from build123d import *

# Parameters (mm, degrees)
SKETCH_1_W          = 42
SKETCH_1_H          = 42
SKETCH_1_R          = 1.5
EXTRUDE_1_DEPTH     = 4.2
SKETCH_2_W          = 42
SKETCH_2_H          = 9.5
SKETCH_2_R          = 1.5
EXTRUDE_2_DEPTH     = 12.5
SKETCH_3_R          = 11.25
CUT_EXTRUDE_1_DEPTH = 33.221886971
SKETCH_4_R          = 3
SKETCH_4_R_2        = 1.5
CUT_EXTRUDE_2_DEPTH = 50.838639628
SKETCH_5_R          = 3.5
CUT_EXTRUDE_3_DEPTH = 2
FILLET_2_R          = 1
FILLET_3_R          = 2


with BuildPart() as part:
    # 草图1 → 凸台-拉伸1 (new body)
    with BuildSketch(Plane(origin=(0, 0, 0), x_dir=(1, 0, 0), z_dir=(0, 1, 0))):
        Rectangle(SKETCH_1_W, SKETCH_1_H)
        with Locations(Location((-15.5, 15.5, 0), (0, 0, 270))):
            Circle(SKETCH_1_R, mode=Mode.SUBTRACT)
        with Locations(Location((15.5, 15.5, 0), (0, 0, 270))):
            Circle(SKETCH_1_R, mode=Mode.SUBTRACT)
        with Locations(Location((-15.5, -15.5, 0), (0, 0, 270))):
            Circle(SKETCH_1_R, mode=Mode.SUBTRACT)
        with Locations(Location((15.5, -15.5, 0), (0, 0, 270))):
            Circle(SKETCH_1_R, mode=Mode.SUBTRACT)
    extrude(amount=EXTRUDE_1_DEPTH)

    # 草图2 → 凸台-拉伸2 (add)
    with BuildSketch(Plane(origin=(0, 4.2, 0), x_dir=(1, 0, 0), z_dir=(0, 1, 0))):
        with Locations((0, 16.25)):
            Rectangle(SKETCH_2_W, SKETCH_2_H)
        with Locations(Location((-15.5, 15.5, 0), (0, 0, 270))):
            Circle(SKETCH_2_R, mode=Mode.SUBTRACT)
        with Locations(Location((15.5, 15.5, 0), (0, 0, 270))):
            Circle(SKETCH_2_R, mode=Mode.SUBTRACT)
    extrude(amount=EXTRUDE_2_DEPTH)

    # 草图3 → 切除-拉伸1 (cut, through all)
    with BuildSketch(Plane(origin=(0, 4.2, 0), x_dir=(1, 0, 0), z_dir=(0, 1, 0))):
        with Locations(Location((0, 0, 0), (0, 0, 270))):
            Circle(SKETCH_3_R)
    extrude(amount=-CUT_EXTRUDE_1_DEPTH, mode=Mode.SUBTRACT)

    # 草图4 → 切除-拉伸2 (cut, through all)
    with BuildSketch(Plane(origin=(0, 0, -21), x_dir=(-1, 0, 0), z_dir=(0, 0, -1))):
        with Locations((-10, 10.7)):
            Circle(SKETCH_4_R)
        with Locations((6, 10.7)):
            Circle(SKETCH_4_R_2)
    extrude(amount=-CUT_EXTRUDE_2_DEPTH, mode=Mode.SUBTRACT)

    # 草图5 → 切除-拉伸3 (cut)
    with BuildSketch(Plane(origin=(0, 0, -21), x_dir=(-1, 0, 0), z_dir=(0, 0, -1))):
        with Locations((6, 10.7)):
            Circle(SKETCH_5_R)
    extrude(amount=-CUT_EXTRUDE_3_DEPTH, mode=Mode.SUBTRACT)

    # 圆角2
    fillet_2_edges = [part.edges().sort_by_distance(p)[0] for p in [
        (21, 2.1, 21),
        (-21, 2.1, 21),
        (-21, 8.35, -21),
        (21, 8.35, -21),
    ]]
    fillet(fillet_2_edges, radius=FILLET_2_R)

    # 圆角3
    fillet_3_edges = [part.edges().sort_by_distance(p)[0] for p in [
        (-21, 10.45, -11.5),
        (21, 10.45, -11.5),
    ]]
    fillet(fillet_3_edges, radius=FILLET_3_R)


solid = part.part
Here's how the part is built. I have some questions about the finished solid (model axes, mm). A direction names the side the tool comes from. Round coordinates to 2 decimals unless told otherwise and drop trailing zeros. Loops run counter-clockwise (first coordinate to the right, second up) from the corner with the lowest first, then second, coordinate; pieces in that order, holes last. Notation, with made-up numbers: M 53.5,-8.5 L 72.5,-8.5 A25 ccw 72.5,3.5 Z; hole C 87.25,-14 d7. An arc over 180 degrees is marked long. Write each question's results on one line, items separated by ' | '. Start each with the question number.
(1) I want a section at D-D (z = 15.5). Please give me the cut outline in (x, y).
(2) I want a section at C-C (y = 10.7). Please give me the cut outline in (x, z).
(3) On a 3-axis mill with a long thin cutter (end or side, diameter ignored), from which of +Z, -Z, +X, -X, +Y, -Y can I reach the whole of each face in a straight line? I mean faces 1 (the cylindrical face through (15.57, 2.07, 14)), 2 (the flat face through (0, 10, -11.5)), 3 (the cylindrical face through (-20.43, 10.54, -12.1)), 4 (the flat face through (-21, 3, -6)), 5 (the flat face through (-6, 9, -19)). Say none if no direction works.
(4) Will these pins go through, and if not, where does the flat tip stop? P1, Ø10, axis at x = 3.5, y = 9, coming from the +Z side; P2, Ø2.5, axis at x = 15.5, z = 15.5, coming from the -Y side; P3, Ø1.5, axis at y = 10, z = -11, coming from the -X side; P4, Ø3.5, axis at x = -6.5, y = 12, coming from the -Z side.
(5) I want a section at A-A (z = -15.5). Please give me the cut outline in (x, y), then the cut area to 3 significant figures.
(6) If I drill on probe 1 along X at (y, z) = (3.05, 15.5); probe 2 along Y at (x, z) = (10, -15); probe 3 along Y at (x, z) = (17, 2), over which ranges is the centre line in solid material (lowest first)? Write a range as from..to.
(7) I want a section at B-B (x = 15.5). Please give me the cut outline in (y, z), then the cut area to 3 significant figures.
(8) Thinking about a two-plate mould opening in Z: for faces 6 (the cylindrical face through (-5.675, 9.236, -15.302)), 7 (the cylindrical face through (20.4, 10.54, -12.07)), 8 (the flat face through (0, 8, -21)), 9 (the cylindrical face through (15.57, 8.23, -17)), which applies, pulls with the +Z half, pulls with the -Z half, needs draft (parallel to the pull), parting line crosses it, or undercut?
Solved:
1) outline: M -21,0 L -17,0 L -17,4.2 L -21,4.2 Z; M -14,0 L 14,0 L 14,4.2 L -14,4.2 Z; M 17,0 L 21,0 L 21,4.2 L 17,4.2 Z
2) outline: M -21,-20 A1 ccw -20,-21 L -9.5,-21 L -9.5,-19 L -7.5,-19 L -7.5,-11.5 L -19,-11.5 A2 ccw -21,-13.5 Z; M -4.5,-19 L -2.5,-19 L -2.5,-21 L 7,-21 L 7,-11.5 L -4.5,-11.5 Z; M 13,-21 L 20,-21 A1 ccw 21,-20 L 21,-13.5 A2 ccw 19,-11.5 L 13,-11.5 Z; hole C -15.5,-15.5 d3; hole C 15.5,-15.5 d3
3) face 1: +Y, -Y | face 2: +Z, +X, -X, +Y | face 3: +Z, -X, +Y | face 4: +Z, -Z, -X, +Y, -Y | face 5: -Z
4) P1: stops at z = 21 | P2: passes through | P3: stops at x = -19.97 | P4: stops at z = -19
5) outline: M -21,0 L -17,0 L -17,16.7 L -21,16.7 Z; M -14,0 L 14,0 L 14,16.7 L -14,16.7 Z; M 17,0 L 21,0 L 21,16.7 L 17,16.7 Z; hole C -6,10.7 d3; hole C 10,10.7 d6 | area: 566 mm²
6) probe 1: x = -21..-17, -14..14, 17..21 | probe 2: y = 0..7.7, 13.7..16.7 | probe 3: y = 0..4.2
7) outline: M 0,-21 L 16.7,-21 L 16.7,-17 L 0,-17 Z; M 0,-14 L 16.7,-14 L 16.7,-11.5 L 4.2,-11.5 L 4.2,14 L 0,14 Z; M 0,17 L 4.2,17 L 4.2,21 L 0,21 Z | area: 232 mm²
8) face 6: needs draft | face 7: pulls with the +Z half | face 8: pulls with the -Z half | face 9: undercut
